Check sheet for the modelled part. Datum: model origin and axes. Units: mm. A direction names the side the tool comes from. Give positions to 0.01 mm unless a question says otherwise; leave off trailing zeros. Loops run counter-clockwise (first coordinate to the right, second up) from the corner with the lowest first, then second, coordinate; pieces in that order, holes last. Notation, with made-up numbers: (18.5, 28) - (42.5, 28) arc R11 ccw to (42.5, 42) - close; hole circle Ø2 at (53, 67). An arc over 180 degrees is marked (long way). Answer in a Markdown table with one row per item. Add a question column.
(1) Sectioned sample at A-A on y = -954.5. Enter the section's corners in (x, z), then the cut area to 3 significant figures.
(2) Sectioned sample at C-C on z = 364.5. Enter the section's corners in (x, y), then the cut area to 3 significant figures.
(3) Draft check along X on faces 3 (the face through (-176.6, -950, 320)), 4 (the face through (-225, -950, 320)), 5 (the face through (-200, -975, 320)). Enter one of: released by +X, released by -X, zero draft, split by the parting line, or undercut.
(4) Sectioned sample at B-B on x = -204. Enter the section's corners in (y, z).
(5) Thickness scan on L1, parallel to Y at x = -214, z = 256.5; L2, parallel to X at y = -938.5, z = 233. Record the ranges inside material, lowest first.
(6) Set-up check for faces 1 (the face through (-202, -974, 650)), 2 (the face through (-200, -973.4, 320)): record each of +Z, -Z, +X, -X, +Y, -Y from which the full face is reachable in a straight line by a thin tool's end or side.
Autodesk Inventor part; units mm, degrees
ref_plane "YZ Plane" through (0, 0, 0) normal (1, 0, 0) x (0, 1, 0)
ref_plane "XZ Plane" through (0, 0, 0) normal (0, 1, 0) x (-1, 0, 0)
ref_plane "XY Plane" through (0, 0, 0) normal (0, 0, 1) x (1, 0, 0)
ref_plane "Work Plane1" through (0, 0, 0) normal (0, 0, 1) x (1, 0, 0)
sketch "Sketch1" plane through (0, 0, 0) normal (0, 0, 1) x (1, 0, 0)
  line L0 (-250, -1000) -> (250, -1000)
  line L1 (250, -1000) -> (250, 1000)
  line L2 (250, 1000) -> (-250, 1000)
  line L3 (-250, 1000) -> (-250, -1000)
  line L4 (-223, -975) -> (-177, -975)
  line L5 (-175, -973) -> (-175, -927)
  line L6 (-177, -925) -> (-223, -925)
  line L7 (-225, -927) -> (-225, -973)
  arc A0 (-225, -973) -> (-223, -975) centre (-223, -973) ccw
  arc A1 (-223, -925) -> (-225, -927) centre (-223, -927) ccw
  arc A2 (-177, -975) -> (-175, -973) centre (-177, -973) ccw
  arc A3 (-175, -927) -> (-177, -925) centre (-177, -927) ccw
  line L8 (-223.4, -973) -> (-223.4, -927)
  arc A4 (-223, -926.6) -> (-223.4, -927) centre (-223, -927) ccw
  line L9 (-223, -926.6) -> (-177, -926.6)
  arc A5 (-176.6, -927) -> (-177, -926.6) centre (-177, -927) ccw
  line L10 (-176.6, -927) -> (-176.6, -973)
  arc A6 (-177, -973.4) -> (-176.6, -973) centre (-177, -973) ccw
  line L11 (-177, -973.4) -> (-223, -973.4)
  arc A7 (-223.4, -973) -> (-223, -973.4) centre (-223, -973) ccw
  point P0 (0, 0)
  point P1 (-175, -925)
  point P2 (-225, -925)
  dimension "d0" = 50
  dimension "d1" = 25
  dimension "d2" = 25
  dimension "d3" = 2
  dimension "d4" = 1.6
extrude "Extrusion1" add sketch "Sketch1" along normal blind 650 contours A0 L7 A1 L6 A3 L5 A2 L4
properties part number "Pata"
Reply:
| question | item | result |
|---|---|---|
| 1 | outline | (-225, 0) - (-223.4, 0) - (-223.4, 650) - (-225, 650) - close; (-176.6, 0) - (-175, 0) - (-175, 650) - (-176.6, 650) - close |
| 1 | area | 2,080 mm^2 |
| 2 | outline | (-225, -973) arc R2 ccw to (-223, -975) - (-177, -975) arc R2 ccw to (-175, -973) - (-175, -927) arc R2 ccw to (-177, -925) - (-223, -925) arc R2 ccw to (-225, -927) - close; hole (-223.4, -973) arc R0.4 ccw to (-223, -973.4) - (-177, -973.4) arc R0.4 ccw to (-176.6, -973) - (-176.6, -927) arc R0.4 ccw to (-177, -926.6) - (-223, -926.6) arc R0.4 ccw to (-223.4, -927) - close |
| 2 | area | 306 mm^2 |
| 3 | face 3 | undercut |
| 3 | face 4 | released by -X |
| 3 | face 5 | zero draft |
| 4 | outline | (-975, 0) - (-973.4, 0) - (-973.4, 650) - (-975, 650) - close; (-926.6, 0) - (-925, 0) - (-925, 650) - (-926.6, 650) - close |
| 5 | L1 | -975 to -973.4, -926.6 to -925 |
| 5 | L2 | -225 to -223.4, -176.6 to -175 |
| 6 | face 1 | +Z, +X, -X, +Y, -Y |
| 6 | face 2 | +Z, -Z |
